Part model, mm, in its own coordinate system. Round coordinates to 2 decimals unless told otherwise and drop trailing zeros. Write each loop counter-clockwise with the first axis right and the second up, starting at its lowest first coordinate (ties: lowest second). Pieces come first, ordered by that corner, then holes. Notation, with made-up numbers: (25.5, 53.5) -> (69.5, 53.5) arc R13 ccw to (69.5, 68.5) -> close; hole circle Ø2 at (71.25, -19.75). An arc over 180 degrees is marked (long way). Use CSV: the item, a comma, the result in double quotes. Start each with the question number.
(1) Probe line 1 (Y direction, x = 0, z = 69); line 2 (X direction, y = 0, z = 75); line 3 (Z direction, x = 40, y = 28). List the from-to ranges inside material, lowest first. Write a range as [from, to].
(2) Two-plate mould, pull along X, no slides. Class faces 1 (the cylindrical face through (1.334, 51.891, 93.722)), 2 (the cylindrical face through (60.57, 0.75, 19.07)), 3 (the cylindrical face through (16.046, 25.167, 73.348)), 4 (the flat face through (-95.25, -1, -1)): released by +X, released by -X, zero draft, split by the parting line, or undercut.
(3) Saw through at A-A (y = 0). Give the cut face in (x, z), plus the area to 3 significant figures.
(4) Saw through at B-B (z = 0). Give the cut face in (x, y), plus the area to 3 significant figures.
(5) Saw through at C-C (x = 0). Give the cut face in (y, z).
(6) Saw through at D-D (z = 29). Give the cut face in (x, y).
```python
from build123d import *

# Parameters (mm, degrees)
F0_W     = 190.5
F0_H     = 190.5
F0_R     = 63.5
F1_DEPTH = 53.34
F2_R     = 29.847135
F3_DEPTH = 190.501
F4_R     = 5.08


with BuildPart() as f1:
    # F0 (on Front) → F1 (new body, symmetric)
    with BuildSketch(Plane.XZ):
        Rectangle(F0_W, F0_H)
        Circle(F0_R, mode=Mode.SUBTRACT)
    extrude(amount=F1_DEPTH, both=True)

    # F2 (on face) → F3 (cut, through all)
    with BuildSketch(Plane.XY.offset(95.25)):
        Circle(F2_R)
    extrude(amount=-F3_DEPTH, mode=Mode.SUBTRACT)

    # F4
    f4_edges = [f1.edges().sort_by_distance(p)[0] for p in [
        (-29.847135, 0, 95.25),
        (0, 53.34, 95.25),
    ]]
    fillet(f4_edges, radius=F4_R)


solid = f1.part
```
Answers:
1,line 1,"y = [-53.34, -29.85], [29.85, 53.34]"
1,line 2,"x = [-95.25, -29.85], [29.85, 95.25]"
1,line 3,"z = [-95.25, -49.32], [49.32, 95.25]"
2,face 1,"zero draft"
2,face 2,"undercut"
2,face 3,"undercut"
2,face 4,"released by -X"
3,outline,"(-95.25, -95.25) -> (-29.85, -95.25) -> (-29.85, -56.05) arc R63.5 cw to (-29.85, 56.05) -> (-29.85, 90.17) arc R5.08 ccw to (-34.93, 95.25) -> (-95.25, 95.25) -> close; (29.85, -95.25) -> (95.25, -95.25) -> (95.25, 95.25) -> (34.93, 95.25) arc R5.08 ccw to (29.85, 90.17) -> (29.85, 56.05) arc R63.5 cw to (29.85, -56.05) -> close"
3,area,"19,500 mm²"
4,outline,"(-95.25, -53.34) -> (-63.5, -53.34) -> (-63.5, 53.34) -> (-95.25, 53.34) -> close; (63.5, -53.34) -> (95.25, -53.34) -> (95.25, 53.34) -> (63.5, 53.34) -> close"
4,area,"6,770 mm²"
5,outline,"(-53.34, -95.25) -> (-29.85, -95.25) -> (-29.85, -63.5) -> (-53.34, -63.5) -> close; (-53.34, 63.5) -> (-29.85, 63.5) -> (-29.85, 90.17) arc R5.08 ccw to (-34.93, 95.25) -> (-53.34, 95.25) -> close; (29.85, -95.25) -> (53.34, -95.25) -> (53.34, -63.5) -> (29.85, -63.5) -> close; (29.85, 63.5) -> (53.34, 63.5) -> (53.34, 90.17) arc R5.08 ccw to (48.26, 95.25) -> (34.93, 95.25) arc R5.08 ccw to (29.85, 90.17) -> close"
6,outline,"(-95.25, -53.34) -> (-56.49, -53.34) -> (-56.49, 53.34) -> (-95.25, 53.34) -> close; (56.49, -53.34) -> (95.25, -53.34) -> (95.25, 53.34) -> (56.49, 53.34) -> close"
